Solid Edge part; units mm, degrees
sketch "Sketch1" plane through (0, 0, 0) normal (0, -1, 0) x (1, 0, 0)
  circle A0 centre (0, 0) radius 4.66
extrude "Protrusion1" add sketch "Sketch1" along normal mid plane 30
sketch "Sketch2" plane through (0, -15, 0) normal (0, -1, 0) x (1, 0, 0)
  circle A0 centre (0, 0) radius 3.5
extrude "ExtrudedProtrusion_2" add sketch "Sketch2" along normal blind 8
hole "Hole_1" at (0, 15, 0) direction (0, -1, 0) diameter 5 depth 35
fillet "Round_1" radius 0.5 3 edges at (-4.66, 15, 0) (0, 15, -2.5) (-3.5, -23, 0)
fillet "Round_2" radius 0.2 2 edges at (-3.5, -15, 0) (-4.66, -15, 0)
Here's how the part is built. I have some questions about the finished solid (model axes, mm). A direction names the side the tool comes from. Give positions to 0.01 mm unless a question says otherwise; leave off trailing zeros. Order: outer loops, then holes, each group sorted by start corner. A loop starts at its lowest first (then second) coordinate and runs counter-clockwise, first axis right, second up. Notation, with made-up numbers: (26.5, -37) - (75.5, -37) arc R37 cw to (75.5, 0) - close; hole circle Ø2 at (-18, 68). An arc over 180 degrees is marked (long way). Answer as a JSON object with one key per item and string values. Group by question number.
Item 1: If we section it at C-C on z = 0: Please give me the cut outline in (x, y), and give its area (3 significant figures).
Item 2: For P1, Ø3, axis at x = -3.5, y = -8, coming from the -Z side; P2, Ø4, axis at x = 3, y = -12.5, coming from the -Z side; P3, Ø1.5, axis at x = -0.5, z = -1, coming from the +Y side, each with a flat end and sliding along its axis, tell me the tip position at first contact or that it passes through.
Item 3: If we section it at D-D on y = -20.5: Please give me the cut outline in (x, z), and give its area (3 significant figures).
Item 4: If we mould it in two halves opening along X, with no side actions, what happens to faces 1 (the cylindrical face through (-3.698, -0.355, -2.836)), 2 (the cylindrical face through (2.44, -2.99, -0.54)), 3 (the flat face through (0, -23, 0))? For each: pulls with the +X half, pulls with the -X half, needs draft (parallel to the pull), parting line crosses it, or undercut.
Item 5: Which directions (+Z, -Z, +X, -X, +Y, -Y) give clear straight access to the entire face, cutting with the end or side of a thin tool? Please do faces 4 (the flat face through (-3, 15, -1)), 5 (the flat face through (4, -15, -1)), 6 (the flat face through (0, -20, 0)).
Item 6: If we section it at B-B on y = -14: Please give me the cut outline in (x, z).
Item 7: Please list where these lines run through material, in increasing order: probe 1 along Z at (x, y) = (0, -2); probe 2 along Y at (x, z) = (1, 0.25); probe 3 along Y at (x, z) = (-1.75, -3.5).
Item 8: If we section it at A-A on x = 0: Please give me the cut outline in (y, z).
Result set:
{
 "1": {"outline": "(-4.66, -14.8) arc R0.2 ccw to (-4.46, -15) - (-3.7, -15) arc R0.2 cw to (-3.5, -15.2) - (-3.5, -22.5) arc R0.5 ccw to (-3, -23) - (3, -23) arc R0.5 ccw to (3.5, -22.5) - (3.5, -15.2) arc R0.2 cw to (3.7, -15) - (4.46, -15) arc R0.2 ccw to (4.66, -14.8) - (4.66, 14.5) arc R0.5 ccw to (4.16, 15) - (3, 15) arc R0.5 ccw to (2.5, 14.5) - (2.5, -20) - (-2.5, -20) - (-2.5, 14.5) arc R0.5 ccw to (-3, 15) - (-4.16, 15) arc R0.5 ccw to (-4.66, 14.5) - close", "area": "160 mm²"},
 "2": {"P1": "z = -4.21", "P2": "z = -4.55", "P3": "y = -20"},
 "3": {"outline": "circle Ø7 at (0, 0)", "area": "38.5 mm²"},
 "4": {"face 1": "parting line crosses it", "face 2": "undercut", "face 3": "needs draft"},
 "5": {"face 4": "+Z, -Z, +X, -X, +Y", "face 5": "-Y", "face 6": "+Y"},
 "6": {"outline": "circle Ø9.32 at (0, 0); hole circle Ø5 at (0, 0)"},
 "7": {"probe 1": "-4.66 to -2.5, 2.5 to 4.66", "probe 2": "-23 to -20", "probe 3": "-15 to 15"},
 "8": {"outline": "(-23, -3) arc R0.5 ccw to (-22.5, -3.5) - (-15.2, -3.5) arc R0.2 cw to (-15, -3.7) - (-15, -4.46) arc R0.2 ccw to (-14.8, -4.66) - (14.5, -4.66) arc R0.5 ccw to (15, -4.16) - (15, -3) arc R0.5 ccw to (14.5, -2.5) - (-20, -2.5) - (-20, 2.5) - (14.5, 2.5) arc R0.5 ccw to (15, 3) - (15, 4.16) arc R0.5 ccw to (14.5, 4.66) - (-14.8, 4.66) arc R0.2 ccw to (-15, 4.46) - (-15, 3.7) arc R0.2 cw to (-15.2, 3.5) - (-22.5, 3.5) arc R0.5 ccw to (-23, 3) - close"}
}
